from build123d import *

# Parameters (mm, degrees)
SKETCH_1_W          = 91
SKETCH_1_H          = 42
EXTRUDE_1_DEPTH     = 5
SKETCH_2_R          = 1.75
SKETCH_2_R_2        = 2.25
CUT_EXTRUDE_1_DEPTH = 5


with BuildPart() as part:
    # 스케치1 → 보스-돌출1 (new body)
    with BuildSketch(Plane(origin=(0, 0, 0), x_dir=(1, 0, 0), z_dir=(0, 1, 0))):
        with Locations((45.5, 21)):
            Rectangle(SKETCH_1_W, SKETCH_1_H)
    extrude(amount=EXTRUDE_1_DEPTH)

    # 스케치2 → 컷-돌출1 (cut)
    with BuildSketch(Plane(origin=(0, 5, 0), x_dir=(1, 0, 0), z_dir=(0, 1, 0))):
        with Locations(Location((28, 33.5, 0), (0, 0, 270))):
            Circle(SKETCH_2_R)
        with Locations(Location((28, 8.5, 0), (0, 0, 270))):
            Circle(SKETCH_2_R)
        with Locations(Location((8, 8.5, 0), (0, 0, 270))):
            Circle(SKETCH_2_R)
        with Locations(Location((8, 33.5, 0), (0, 0, 270))):
            Circle(SKETCH_2_R)
        with Locations(Location((42.094873015, 28, 0), (0, 0, 270))):
            Circle(SKETCH_2_R_2)
        with Locations(Location((42.094873015, 14, 0), (0, 0, 270))):
            Circle(SKETCH_2_R_2)
        with Locations(Location((84.094873015, 14, 0), (0, 0, 270))):
            Circle(SKETCH_2_R_2)
        with Locations(Location((84.094873015, 28, 0), (0, 0, 270))):
            Circle(SKETCH_2_R_2)
    extrude(amount=-CUT_EXTRUDE_1_DEPTH, mode=Mode.SUBTRACT)


solid = part.part
Design review of the part built by this model. Coordinates are the model's own, in mm. Round coordinates to 2 decimals unless told otherwise and drop trailing zeros. Write each loop counter-clockwise with the first axis right and the second up, starting at its lowest first coordinate (ties: lowest second). Pieces come first, ordered by that corner, then holes.
Item 1: Draft analysis for pull direction X (two halves, no side actions). For faces 1 (the flat face through (45, 5, -21)), 2 (the flat face through (0, 2, -21)), 3 (the cylindrical face through (9.18, 2.54, -34.79)), 4 (the cylindrical face through (9.5, 2.5, -7.6)), state which applies: released by +X, released by -X, zero draft, split by the parting line, or undercut.
Item 2: For pin 1 Ø4.5 at (x, z) = (28, -8.5) entering from -Y, flat-tipped, find the tip position at first contact; note if it passes through.
Item 3: Consider section B-B on z = -28. Give the boundary of the cut face in (x, y), and give its area (3 significant figures).
Item 4: Wall thickness on L1, parallel to X at y = 3.15, z = -8.5; L2, parallel to X at y = 3.6, z = -14; L3, parallel to Z at x = 8.5, y = 2.8: over which ranges is each line inside the solid? List them lowest first.
Item 5: Consider section A-A on x = 8. Give the boundary of the cut face in (y, z), and give its area (3 significant figures).
Item 6: Consider section C-C on y = 1.1. Count the separate pieces of the cut face and the enclosed holes in it, and give its area (3 significant figures).
Check values:
1. face 1: zero draft
1. face 2: released by -X
1. face 3: undercut
1. face 4: undercut
2. pin 1: stops at y = 0
3. outline: (0, 0) - (39.84, 0) - (39.84, 5) - (0, 5) - close; (44.34, 0) - (81.84, 0) - (81.84, 5) - (44.34, 5) - close; (86.34, 0) - (91, 0) - (91, 5) - (86.34, 5) - close
3. area: 410 mm2
4. L1: x = 0 to 6.25, 9.75 to 26.25, 29.75 to 91
4. L2: x = 0 to 39.84, 44.34 to 81.84, 86.34 to 91
4. L3: z = -42 to -35.18, -31.82 to -10.18, -6.82 to 0
5. outline: (0, -42) - (5, -42) - (5, -35.25) - (0, -35.25) - close; (0, -31.75) - (5, -31.75) - (5, -10.25) - (0, -10.25) - close; (0, -6.75) - (5, -6.75) - (5, 0) - (0, 0) - close
5. area: 175 mm2
6. separate pieces: 1
6. enclosed holes: 8
6. area: 3,720 mm2
